Read the model definition and answer for the solid it produces. Units are mm, in the model's axes. Give positions to 0.01 mm unless a question says otherwise; leave off trailing zeros. Write each loop counter-clockwise with the first axis right and the second up, starting at its lowest first coordinate (ties: lowest second). Pieces come first, ordered by that corner, then holes. Notation, with made-up numbers: (59.5, 38.5) -> (116.5, 38.5) arc R27 cw to (116.5, 61.5) -> close; hole circle Ø10 at (14, 63). An arc over 180 degrees is marked (long way). Answer as CSV lines item,"result". Start each with the question number.
1. Find the intervals of material crossed by line 1 (X direction, y = 43.5, z = 2.3); line 2 (Y direction, x = 39, z = 4.85); line 3 (Y direction, x = -21.5, z = 1.15), in increasing order.
2. The part is cut by section B-B, the plane y = 6.5. Determine the outline of the cut face in (x, z).
3. The part is cut by section C-C, the plane z = 1.6. Give the number of separate pieces and of enclosed holes in the cut face, and give its area (3 significant figures).
4. The part is cut by section A-A, the plane x = 38.5. Determine the outline of the cut face in (y, z), and give its area (3 significant figures).
5. The part is cut by section D-D, the plane x = -38. Determine the outline of the cut face in (y, z), and give its area (3 significant figures).
6. Given pin 1 (5 mm diameter, centred on x = -20.83, y = 0, fed in from -Z); pin 2 (2.5 mm diameter, centred on y = 0.5, z = 2.5, fed in from -X); pin 3 (1 mm diameter, centred on y = 7, z = 4.5, fed in from -X); pin 4 (1 mm diameter, centred on x = -30, z = 1.5, fed in from -Y), each flat-ended and moving along its own axis, determine where each tip first touches the part or whether it passes through.
from build123d import *

# Parameters (mm, degrees)
F1_DEPTH = 5.08
F2_R     = 4


# Not quite as in the source:
# - a feature names something its author has since deleted; it is built from what else it names


with BuildPart() as f1:
    # F0 (on Top) → F1 (new body)
    with BuildSketch(Plane.XY):
        with BuildLine():
            Line((0.6656670719, 55.8519247654), (-50.5843329281, 55.8519247654))
            ThreePointArc((-50.5843329281, 55.8519247654), (-50.7903791398, 55.0931866065), (-51.3519110531, 54.5428952787))
            Line((-51.3519110531, 54.5428952787), (-49.566514597, 51.3519247654))
            Line((-49.566514597, 51.3519247654), (-11.1088099211, 51.3519247654))
            Line((-11.1088099211, 51.3519247654), (-3.1543997556, 51.3519247654))
            Line((-3.1543997556, 51.3519247654), (5.4156670719, 51.3519247654))
            Line((5.4156670719, 51.3519247654), (10.9156670719, 51.3519247654))
            Line((10.9156670719, 51.3519247654), (10.9156670719, 55.8519247654))
            Line((10.9156670719, 55.8519247654), (3.6656670719, 55.8519247654))
            ThreePointArc((3.6656670719, 55.8519247654), (2.1656670719, 54.3519247654), (0.6656670719, 55.8519247654))
        make_face()
        with BuildLine():
            Line((-11.1088099211, 4.5), (-23.3521512592, 4.5))
            Line((-23.3521512592, 4.5), (-21.5667548031, 1.3090294867))
            ThreePointArc((-21.5667548031, 1.3090294867), (-20.0755947692, 1.2939537883), (-19.3343329281, 0))
            Line((-19.3343329281, 0), (10.9156670719, 0))
            Line((10.9156670719, 0), (10.9156670719, 4.5))
            Line((10.9156670719, 4.5), (5.4156670719, 4.5))
            Line((5.4156670719, 4.5), (-3.1543997556, 4.5))
            Line((-3.1543997556, 4.5), (-11.1088099211, 4.5))
        make_face()
        with BuildLine():
            ThreePointArc((-51.3519110531, 54.5428952787), (-53.3782867164, 56.6106629243), (-50.5843329281, 55.8519247654))
            Line((-50.5843329281, 55.8519247654), (0.6656670719, 55.8519247654))
            ThreePointArc((0.6656670719, 55.8519247654), (2.1656670719, 57.3519247654), (3.6656670719, 55.8519247654))
            Line((3.6656670719, 55.8519247654), (10.9156670719, 55.8519247654))
            Line((10.9156670719, 55.8519247654), (18.1656670719, 55.8519247654))
            ThreePointArc((18.1656670719, 55.8519247654), (19.6656670719, 57.3519247654), (21.1656670719, 55.8519247654))
            Line((21.1656670719, 55.8519247654), (71.6656670719, 55.8519247654))
            ThreePointArc((71.6656670719, 55.8519247654), (73.9156670719, 58.1019247654), (76.1656670719, 55.8519247654))
            ThreePointArc((76.1656670719, 55.8519247654), (75.0537743102, 53.910994083), (72.8170342594, 53.8883805354))
            Line((72.8170342594, 53.8883805354), (71.3978487408, 51.3519247654))
            Line((71.3978487408, 51.3519247654), (81.8841302488, 51.3519247654))
            Line((81.8841302488, 51.3519247654), (81.8841302488, 60.3519247654))
            Line((81.8841302488, 60.3519247654), (-60.052796105, 60.3519247654))
            Line((-60.052796105, 60.3519247654), (-60.052796105, 51.3519247654))
            Line((-60.052796105, 51.3519247654), (-49.566514597, 51.3519247654))
            Line((-49.566514597, 51.3519247654), (-51.3519110531, 54.5428952787))
        make_face()
        with BuildLine():
            Line((-21.5667548031, 1.3090294867), (-23.3521512592, 4.5))
            Line((-23.3521512592, 4.5), (-27.3365851734, 4.5))
            Line((-27.3365851734, 4.5), (-27.3365851734, -4.5))
            Line((-27.3365851734, -4.5), (49.1679193172, -4.5))
            Line((49.1679193172, -4.5), (49.1679193172, 4.5))
            Line((49.1679193172, 4.5), (45.183485403, 4.5))
            Line((45.183485403, 4.5), (43.3980889469, 1.3090294867))
            ThreePointArc((43.3980889469, 1.3090294867), (43.9596208602, 0.7587381589), (44.1656670719, 0))
            ThreePointArc((44.1656670719, 0), (42.6656670719, -1.5), (41.1656670719, 0))
            Line((41.1656670719, 0), (31.1806510627, 0))
            Line((31.1806510627, 0), (31.1806510627, -2.5))
            Line((31.1806510627, -2.5), (28.0056510627, -2.5))
            Line((28.0056510627, -2.5), (28.0056510627, 0))
            Line((28.0056510627, 0), (19.9686510627, 0))
            Line((19.9686510627, 0), (19.9686510627, -2.5))
            Line((19.9686510627, -2.5), (16.7936510627, -2.5))
            Line((16.7936510627, -2.5), (16.7936510627, 0))
            Line((16.7936510627, 0), (10.9156670719, 0))
            Line((10.9156670719, 0), (-19.3343329281, 0))
            ThreePointArc((-19.3343329281, 0), (-21.593071087, -1.2939537883), (-21.5667548031, 1.3090294867))
        make_face()
        with BuildLine():
            Line((10.9156670719, 4.5), (10.9156670719, 0))
            Line((10.9156670719, 0), (16.7936510627, 0))
            Line((16.7936510627, 0), (16.7936510627, 2.5))
            Line((16.7936510627, 2.5), (19.9686510627, 2.5))
            Line((19.9686510627, 2.5), (19.9686510627, 0))
            Line((19.9686510627, 0), (28.0056510627, 0))
            Line((28.0056510627, 0), (28.0056510627, 2.5))
            Line((28.0056510627, 2.5), (31.1806510627, 2.5))
            Line((31.1806510627, 2.5), (31.1806510627, 0))
            Line((31.1806510627, 0), (41.1656670719, 0))
            ThreePointArc((41.1656670719, 0), (41.906928913, 1.2939537883), (43.3980889469, 1.3090294867))
            Line((43.3980889469, 1.3090294867), (45.183485403, 4.5))
            Line((45.183485403, 4.5), (32.9401440649, 4.5))
            Line((32.9401440649, 4.5), (24.9857338994, 4.5))
            Line((24.9857338994, 4.5), (16.4156670719, 4.5))
            Line((16.4156670719, 4.5), (10.9156670719, 4.5))
        make_face()
        with BuildLine():
            Line((18.1656670719, 55.8519247654), (10.9156670719, 55.8519247654))
            Line((10.9156670719, 55.8519247654), (10.9156670719, 51.3519247654))
            Line((10.9156670719, 51.3519247654), (16.4156670719, 51.3519247654))
            Line((16.4156670719, 51.3519247654), (24.9857338994, 51.3519247654))
            Line((24.9857338994, 51.3519247654), (32.9401440649, 51.3519247654))
            Line((32.9401440649, 51.3519247654), (71.3978487408, 51.3519247654))
            Line((71.3978487408, 51.3519247654), (72.8170342594, 53.8883805354))
            ThreePointArc((72.8170342594, 53.8883805354), (71.9747363894, 54.7138175271), (71.6656670719, 55.8519247654))
            Line((71.6656670719, 55.8519247654), (21.1656670719, 55.8519247654))
            ThreePointArc((21.1656670719, 55.8519247654), (19.6656670719, 54.3519247654), (18.1656670719, 55.8519247654))
        make_face()
        Polygon((5.4156670719, 39.2025500407), (5.4156670719, 27.9259623827), (10.9156670719, 27.9259623827), (10.9156670719, 51.3519247654), (5.4156670719, 51.3519247654), align=None)
        Polygon((10.9156670719, 27.9259623827), (5.4156670719, 27.9259623827), (5.4156670719, 16.6493747247), (5.4156670719, 4.5), (10.9156670719, 4.5), align=None)
        Polygon((16.4156670719, 51.3519247654), (10.9156670719, 51.3519247654), (10.9156670719, 27.9259623827), (16.4156670719, 27.9259623827), (16.4156670719, 39.2025500407), align=None)
        Polygon((16.4156670719, 27.9259623827), (10.9156670719, 27.9259623827), (10.9156670719, 4.5), (16.4156670719, 4.5), (16.4156670719, 16.6493747247), align=None)
        Polygon((-3.1543997556, 51.3519247654), (-11.1088099211, 51.3519247654), (5.4156670719, 27.9259623827), (5.4156670719, 39.2025500407), align=None)
        Polygon((5.4156670719, 27.9259623827), (-11.1088099211, 4.5), (-3.1543997556, 4.5), (5.4156670719, 16.6493747247), align=None)
        Polygon((32.9401440649, 4.5), (16.4156670719, 27.9259623827), (16.4156670719, 16.6493747247), (24.9857338994, 4.5), align=None)
        Polygon((16.4156670719, 39.2025500407), (16.4156670719, 27.9259623827), (32.9401440649, 51.3519247654), (24.9857338994, 51.3519247654), align=None)
    extrude(amount=F1_DEPTH)

    # F2
    f2_edges = [f1.edges().sort_by_distance(p)[0] for p in [
        (-60.052796, 60.351925, 2.54),
        (-60.052796, 51.351925, 2.54),
        (81.88413, 60.351925, 2.54),
        (81.88413, 51.351925, 2.54),
        (49.167919, 4.5, 2.54),
        (49.167919, -4.5, 2.54),
        (-27.336585, 4.5, 2.54),
        (-27.336585, -4.5, 2.54),
    ]]
    fillet(f2_edges, radius=F2_R)


solid = f1.part
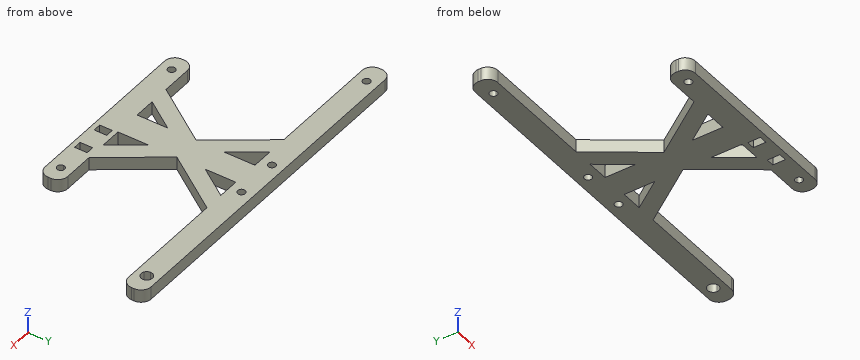
Results found:
1,line 1,"x = -5.57 to 2.38, 5.42 to 16.42, 19.45 to 27.4"
1,line 2,"y = -4.5 to 4.5, 51.35 to 60.35"
1,line 3,"y = -4.5 to -1.34, 1.34 to 4.5, 51.35 to 60.35"
2,outline,"(-9.7, 0) -> (-1.74, 0) -> (-1.74, 5.08) -> (-9.7, 5.08) -> close; (5.42, 0) -> (16.42, 0) -> (16.42, 5.08) -> (5.42, 5.08) -> close; (23.57, 0) -> (31.53, 0) -> (31.53, 5.08) -> (23.57, 5.08) -> close"
3,separate pieces,"1"
3,enclosed holes,"12"
3,area,"2,940 mm²"
4,outline,"(-4.5, 0) -> (4.5, 0) -> (4.5, 5.08) -> (-4.5, 5.08) -> close; (51.35, 0) -> (60.35, 0) -> (60.35, 5.08) -> (51.35, 5.08) -> close"
4,area,"91.4 mm²"
5,outline,"(51.35, 0) -> (60.35, 0) -> (60.35, 5.08) -> (51.35, 5.08) -> close"
5,area,"45.7 mm²"
6,pin 1,"stops at z = 0"
6,pin 2,"stops at x = -27.34"
6,pin 3,"stops at x = -9.7"
6,pin 4,"stops at y = 51.35"
